Geometry check sheet. Reference: the model listing, model coordinates, mm. A direction names the side the tool comes from. Coordinates: 2 decimals unless noted, no trailing zeros. Write each loop counter-clockwise with the first axis right and the second up, starting at its lowest first coordinate (ties: lowest second). Pieces come first, ordered by that corner, then holes. Notation, with made-up numbers: (-26, 54.5) -> (5, 54.5) arc R31 ccw to (5, 78.5) -> close; hole circle Ø5 at (-39.75, 30.25). An arc over 180 degrees is marked (long way). Answer in a Markdown table with one row per item. Add a question column.
Q1. Section check C-C, the plane y = -7.5. Record the boundary of the cut face in (x, z).
Q2. Section check A-A, the plane z = 3.75. Record the boundary of the cut face in (x, y).
Q3. Release check for a two-part mould opening along Y. For faces 4 (the face through (-19.916, -2.801, 2.285)), 5 (the face through (15.301, -1.035, 6.042)), 6 (the face through (28.028, -1.035, 1.699)), 7 (the face through (-0.4, 10, 0.5)) record: pulls with the +Y half, pulls with the -Y half, needs draft (parallel to the pull), parting line crosses it, or undercut.
Q4. Section check B-B, the plane x = -22.5. Record the boundary of the cut face in (y, z).
Q5. Thickness scan on line 1 (Y direction, x = 21, z = 7.5); line 2 (X direction, y = -2, z = 3.5). Record the ranges inside material, lowest first.
Q6. Tool access check on faces 1 (the face through (-15.4, -1.8, 8.8)), 2 (the face through (-24.715, 1.051, 6.042)), 3 (the face through (0.196, 1.051, 1.715)). Record the directions out of +Z, -Z, +X, -X, +Y, -Y that give a thin tool (end or side, any length) a straight path to the whole face; none if there is none.
Q7. Gauge pin test, flat ends, axial feed: P1, Ø8, axis at x = -18.5, y = 3, coming from the +Z side; P2, Ø2, axis at x = -2.5, y = 6, coming from the +Z side; P3, Ø0.8, axis at y = -2, z = 5.5, coming from the -X side; P4, Ø0.6, axis at y = 2, z = 5.5, coming from the +X side. Record the tip position at first contact, or that the pin passes through.
```python
from build123d import *

# Parameters (mm, degrees)
F0_W     = 60
F0_H     = 20
F1_DEPTH = 2
F2_W     = 10
F2_H     = 5
F3_DEPTH = 7
F4_W     = 60
F4_H     = 1.5
F5_DEPTH = 8
F6_F1_R  = 1
F6_F2_R  = 0.9999


# Not quite as in the source:
# - a fillet or chamfer is up to 0.001 mm smaller than in the source, because OpenCascade refuses the exact size


with BuildPart() as f1:
    # F0 (on Top) → F1 (new body)
    with BuildSketch(Plane.XY):
        Rectangle(F0_W, F0_H)
    extrude(amount=F1_DEPTH)

    # F2 (on face) → F3 (join)
    with BuildSketch(Plane.XY.offset(2)):
        with Locations((-20, 0)):
            Rectangle(F2_W, F2_H)
        with Locations((20, 0)):
            Rectangle(F2_W, F2_H)
    extrude(amount=F3_DEPTH)

    # F4 (on face) → F5 (cut)
    with BuildSketch(Plane.XY.offset(9)):
        Rectangle(F4_W, F4_H)
    extrude(amount=-F5_DEPTH, mode=Mode.SUBTRACT)

    # F6: fillet of radius 1 on 32 edges, made by hand

    # F6_f1
    f6_f1_edges = [f1.edges().sort_by_distance(p)[0] for p in [
        (-25, -1.625, 2),
        (-20, -2.5, 2),
        (-15, -1.625, 2),
        (15, -1.625, 2),
        (20, -2.5, 2),
        (25, -1.625, 2),
        (25, 1.625, 2),
        (20, 2.5, 2),
        (15, 1.625, 2),
        (-15, 1.625, 2),
        (-20, 2.5, 2),
        (-25, 1.625, 2),
    ]]
    fillet(f6_f1_edges, radius=F6_F1_R)

    # F6_f2 (radius 1 in the source; OpenCascade refuses exactly that, so slightly less here)
    f6_f2_edges = [f1.edges().sort_by_distance(p)[0] for p in [
        (-15, 1.625, 9),
        (-25, 1.625, 9),
        (-25, -1.625, 9),
        (-15, -1.625, 9),
        (15, 1.625, 9),
        (15, -1.625, 9),
        (25, 1.625, 9),
        (25, -1.625, 9),
        (-28, -0.75, 2),
        (0, -0.75, 2),
        (28, -0.75, 2),
        (30, -5.375, 2),
        (0, -10, 2),
        (-30, -5.375, 2),
        (0, 10, 2),
        (30, 5.375, 2),
        (28, 0.75, 2),
        (0, 0.75, 2),
        (-28, 0.75, 2),
        (-30, 5.375, 2),
        (-25.2928932188, 0.75, 2.2928932188),
        (14.7071067812, 0.75, 2.2928932188),
        (-14.7071067812, 0.75, 2.2928932188),
        (25.2928932188, 0.75, 2.2928932188),
        (25.2928932188, -0.75, 2.2928932188),
        (-14.7071067812, -0.75, 2.2928932188),
        (14.7071067812, -0.75, 2.2928932188),
        (-25.2928932188, -0.75, 2.2928932188),
    ]]
    fillet(f6_f2_edges, radius=F6_F2_R)


solid = f1.part
```
Calculated:
| question | item | result |
|---|---|---|
| 1 | outline | (-30, 0) -> (30, 0) -> (30, 1) arc R1 ccw to (29, 2) -> (-29, 2) arc R1 ccw to (-30, 1) -> close |
| 2 | outline | (-25, -2.5) -> (-15, -2.5) -> (-15, -1.75) arc R1 ccw to (-16, -0.75) -> (-24, -0.75) arc R1 ccw to (-25, -1.75) -> close; (-25, 1.75) arc R1 ccw to (-24, 0.75) -> (-16, 0.75) arc R1 ccw to (-15, 1.75) -> (-15, 2.5) -> (-25, 2.5) -> close; (15, -2.5) -> (25, -2.5) -> (25, -1.75) arc R1 ccw to (24, -0.75) -> (16, -0.75) arc R1 ccw to (15, -1.75) -> close; (15, 1.75) arc R1 ccw to (16, 0.75) -> (24, 0.75) arc R1 ccw to (25, 1.75) -> (25, 2.5) -> (15, 2.5) -> close |
| 3 | face 4 | pulls with the -Y half |
| 3 | face 5 | undercut |
| 3 | face 6 | undercut |
| 3 | face 7 | pulls with the +Y half |
| 4 | outline | (-10, 0) -> (10, 0) -> (10, 1) arc R1 ccw to (9, 2) -> (3.5, 2) arc R1 cw to (2.5, 3) -> (2.5, 9) -> (0.75, 9) -> (0.75, 1) -> (-0.75, 1) -> (-0.75, 9) -> (-2.5, 9) -> (-2.5, 3) arc R1 cw to (-3.5, 2) -> (-9, 2) arc R1 ccw to (-10, 1) -> close |
| 5 | line 1 | y = -2.5 to -0.75, 0.75 to 2.5 |
| 5 | line 2 | x = -25 to -15, 15 to 25 |
| 6 | face 1 | +Z, +Y, -Y |
| 6 | face 2 | +Z, -X |
| 6 | face 3 | +Z |
| 7 | P1 | stops at z = 9 |
| 7 | P2 | stops at z = 2 |
| 7 | P3 | stops at x = -25 |
| 7 | P4 | stops at x = 25 |
